Autodesk Inventor part; units mm, degrees
ref_plane "YZ Plane" through (0, 0, 0) normal (1, 0, 0) x (0, 1, 0)
ref_plane "XZ Plane" through (0, 0, 0) normal (0, 1, 0) x (-1, 0, 0)
ref_plane "XY Plane" through (0, 0, 0) normal (0, 0, 1) x (1, 0, 0)
sketch "Sketch1" plane through (0, 0, 0) normal (0, 1, 0) x (-1, 0, 0)
  circle A0 centre (7.7, 5.2) radius 1.5
  circle A1 centre (7.7, -5.2) radius 1.5
  circle A2 centre (0, 0) radius 1.5
  line L0 (37.8003, -0.0084) -> (-30.1744, -0.0084) construction
  line L1 (-27.0022, -36.8848) -> (-27.0022, -0.0084)
  line L2 (12.164, -30.8563) -> (6.1355, -36.8848)
  line L3 (-27.0022, -36.8848) -> (6.1355, -36.8848)
  line L4 (36.1543, -0.0084) -> (36.1543, -17.0084)
  line L5 (36.1543, -17.0084) -> (12.164, -30.8563)
  line L6 (-27.0022, 36.8681) -> (-27.0022, -0.0084)
  line L7 (12.164, 30.8396) -> (6.1355, 36.8681)
  line L8 (-27.0022, 36.8681) -> (6.1355, 36.8681)
  line L9 (36.1543, -0.0084) -> (36.1543, 16.9916)
  line L10 (36.1543, 16.9916) -> (12.164, 30.8396)
extrude "Extrusion1" add sketch "Sketch1" along normal blind 3
sketch "Sketch2" plane through (0, 3, 0) normal (0, 1, 0) x (1, 0, 0)
  circle A0 centre (13, 13.115) radius 3.5
  point P0 (0, 0)
  dimension "d2" = 7
  dimension "d3" = 13.115
  dimension "d4" = 13
extrude "Extrusion2" cut sketch "Sketch2" against normal through all
move faces "Move1" translate (0.9995, 0, 0) faces at (27.0022, 1, -12.3005)
sketch "Sketch5" plane through (0, 0, 0) normal (0, -1, 0) x (1, 0, 0)
  circle A0 centre (18.0046, -22.074) radius 1.5
  circle A1 centre (8.0046, -22.0753) radius 1.5
  circle A2 centre (17.9981, 27.7053) radius 1.5
  circle A3 centre (7.9981, 27.704) radius 1.5
  line L0 (22.8987, 23.1163) -> (22.904, -17.4837)
  line L1 (22.904, -17.4837) -> (3.104, -17.4863)
  line L2 (3.0987, 23.1137) -> (22.8987, 23.1163)
  line L3 (3.104, -17.4863) -> (3.0987, 23.1137)
  point P0 (0, 0)
extrude "Extrusion4" cut sketch "Sketch5" against normal through all
sketch "Sketch6" plane through (0, 3, 0) normal (0, 1, 0) x (1, 0, 0)
  circle A0 centre (0, 0) radius 1.5
  circle A1 centre (26.6, 0) radius 1.5
  dimension "d22" = 3
  dimension "d23" = 26.6
move faces "Move2" translate (3.9857, 0, 0) faces at (28.0017, 1, -12.3005)
extrude "Extrusion5" cut sketch "Sketch6" against normal through all
sketch "Sketch7" plane through (0, 3, 0) normal (0, 1, 0) x (1, 0, 0)
  line L0 (27.9874, -33.8681) -> (19.9874, -33.8681)
  line L1 (19.9874, -30.8681) -> (19.9874, -33.8681)
  line L2 (27.9874, -30.8681) -> (27.9874, -33.8681)
  line L3 (19.9874, -30.8681) -> (27.9874, -30.8681)
  line L4 (5.8645, -33.8681) -> (-2.1355, -33.8681)
  line L5 (-2.1355, -30.8681) -> (-2.1355, -33.8681)
  line L6 (-2.1355, -30.8681) -> (5.8645, -30.8681)
  line L7 (5.8645, -30.8681) -> (5.8645, -33.8681)
  line L8 (-2.1355, 32.1319) -> (5.8645, 32.1319)
  line L9 (5.8645, 29.1319) -> (-2.1355, 29.1319)
  line L10 (5.8645, 32.1319) -> (5.8645, 29.1319)
  line L11 (-2.1355, 32.1319) -> (-2.1355, 29.1319)
  line L12 (19.9874, 32.1319) -> (19.9874, 29.1319)
  line L13 (27.9874, 32.1319) -> (27.9874, 29.1319)
  line L14 (27.9874, 29.1319) -> (19.9874, 29.1319)
  line L15 (19.9874, 32.1319) -> (27.9874, 32.1319)
  point P0 (0, 0)
  point P1 (31.9874, -36.8681)
extrude "Extrusion6" cut sketch "Sketch7" against normal through all
sketch "Sketch8" plane through (0, 3, 0) normal (0, 1, 0) x (1, 0, 0)
  line L0 (5.8645, -33.8681) -> (-2.1355, -33.8681)
  line L1 (-2.1355, -35.8681) -> (-2.1355, -36.8681) construction
  line L2 (-2.1355, 32.1319) -> (5.8645, 32.1319) construction
  line L3 (31.9874, 35.8848) -> (-7.1355, 35.8848)
  line L4 (31.9874, -35.8681) -> (-7.1355, -35.8681)
  line L5 (31.9874, -36.8681) -> (31.9874, -35.8681)
  line L6 (31.9874, 35.8848) -> (31.9874, 36.8848)
  line L7 (-6.1355, 36.8848) -> (-7.1355, 35.8848)
  line L8 (-6.1355, -36.8681) -> (-7.1355, -35.8681)
  line L9 (-6.1355, -36.8681) -> (31.9874, -36.8681)
  line L10 (-6.1355, 36.8848) -> (31.9874, 36.8848)
  point P0 (0, 0)
  dimension "d32" = 2
extrude "Extrusion7" cut sketch "Sketch8" against normal through all
sketch "Sketch9" plane through (0, 3, 0) normal (0, 1, 0) x (1, 0, 0)
  line L0 (-12.164, 30.8563) -> (-12.164, 14.1606) construction
  line L1 (-12.164, 26.3921) -> (-12.164, 30.8563)
  line L2 (-36.1543, 17.0084) -> (-12.164, 30.8563)
  line L3 (-36.1543, 17.0084) -> (-12.164, 30.8563)
  line L4 (-36.1543, 17.0084) -> (-12.164, 26.3921)
  line L5 (-41.6853, 0) -> (0, 0) construction
  line L6 (-12.164, -30.8396) -> (-12.164, -14.1438) construction
  line L7 (-12.164, -26.3753) -> (-12.164, -30.8396)
  line L8 (-36.1543, -16.9916) -> (-12.164, -30.8396)
  line L9 (-36.1543, -16.9916) -> (-12.164, -26.3753)
extrude "Extrusion8" cut sketch "Sketch9" against normal up to next
fillet "Fillet1" radius 6 2 edges at (-7.1355, 1.5, -35.8848) (-7.1355, 1.5, 35.8681)
fillet "Fillet2" radius 2 4 edges at (-12.164, 1.5, -26.3921) (-12.164, 1.5, 26.3753) (-12.164, 1.5, 30.8396) (-12.164, 1.5, -30.8563)
fillet "Fillet3" radius 4 2 edges at (-36.1543, 1.5, 16.9916) (-36.1543, 1.5, -17.0084)
properties part number "Dock bot2" material "Acrylic"
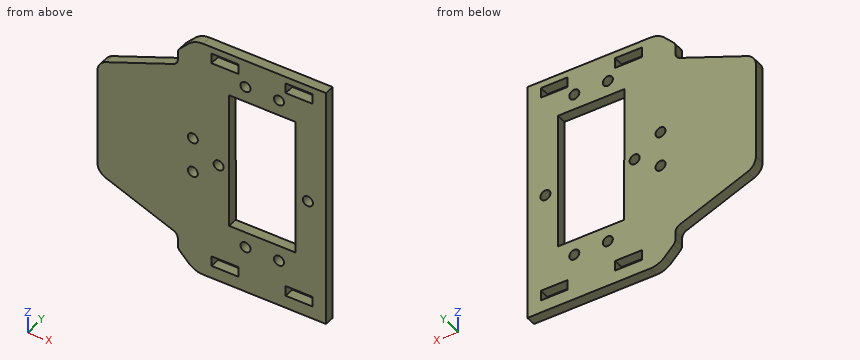
Could you check a few things on this model? Use its own coordinates, in mm. Round coordinates to 2 decimals unless told otherwise and drop trailing zeros. Write each loop counter-clockwise with the first axis right and the second up, starting at its lowest first coordinate (ties: lowest second). Pieces come first, ordered by that corner, then holes. Notation, with made-up numbers: (62, 62.5) -> (78, 62.5) arc R24 ccw to (78, 94.5) -> close; hole circle Ø9 at (71.25, 60). An arc over 180 degrees is marked (long way). Use a Markdown table: item, result.
1. If we section it at A-A (x = 26.6): List the corners of the cut face in (y, z) for me, then the cut area to 3 significant figures.
Answer key:
| item | result |
|---|---|
| outline | (0, -35.88) -> (3, -35.88) -> (3, -32.13) -> (0, -32.13) -> close; (0, -29.13) -> (3, -29.13) -> (3, -1.5) -> (0, -1.5) -> close; (0, 1.5) -> (3, 1.5) -> (3, 30.87) -> (0, 30.87) -> close; (0, 33.87) -> (3, 33.87) -> (3, 35.87) -> (0, 35.87) -> close |
| area | 188 mm^2 |
2. For pin 1 Ø2.5 at (x, z) = (-7.7, 5.2) entering from -Y; pin 2 Ø1.5 at (y, z) = (1.5, 32.5) entering from -X, each with a flat end and sliding along its axis, tell me the tip position at first contact or that it passes through.
Answer key:
| item | result |
|---|---|
| pin 1 | passes through |
| pin 2 | stops at x = -11.25 |
3. If we section it at C-C (z = -13): List the corners of the cut face in (x, y) for me, then the cut area to 3 significant figures.
Answer key:
| item | result |
|---|---|
| outline | (-36.15, 0) -> (3.1, 0) -> (3.1, 3) -> (-36.15, 3) -> close; (22.9, 0) -> (31.99, 0) -> (31.99, 3) -> (22.9, 3) -> close |
| area | 145 mm^2 |
4. Please list where these lines run through material, in increasing order: probe 1 along Z at (x, y) = (21.5, 1.55); probe 2 along Z at (x, y) = (0, 0.95); probe 3 along X at (y, z) = (1.2, 0).
Answer key:
| item | result |
|---|---|
| probe 1 | z = -35.88 to -32.13, -29.13 to -17.48, 23.12 to 30.87, 33.87 to 35.87 |
| probe 2 | z = -35.88 to -32.13, -29.13 to -1.5, 1.5 to 30.87, 33.87 to 35.87 |
| probe 3 | x = -36.15 to -1.5, 1.5 to 3.1, 22.9 to 25.1, 28.1 to 31.99 |
5. If we section it at D-D (x = -7.7): List the corners of the cut face in (y, z) for me.
Answer key:
| item | result |
|---|---|
| outline | (0, -35.05) -> (3, -35.05) -> (3, -6.7) -> (0, -6.7) -> close; (0, -3.7) -> (3, -3.7) -> (3, 3.7) -> (0, 3.7) -> close; (0, 6.7) -> (3, 6.7) -> (3, 35.04) -> (0, 35.04) -> close |
6. If we section it at B-B (z = 0): List the corners of the cut face in (x, y) for me, then the cut area to 3 significant figures.
Answer key:
| item | result |
|---|---|
| outline | (-36.15, 0) -> (-1.5, 0) -> (-1.5, 3) -> (-36.15, 3) -> close; (1.5, 0) -> (3.1, 0) -> (3.1, 3) -> (1.5, 3) -> close; (22.9, 0) -> (25.1, 0) -> (25.1, 3) -> (22.9, 3) -> close; (28.1, 0) -> (31.99, 0) -> (31.99, 3) -> (28.1, 3) -> close |
| area | 127 mm^2 |
